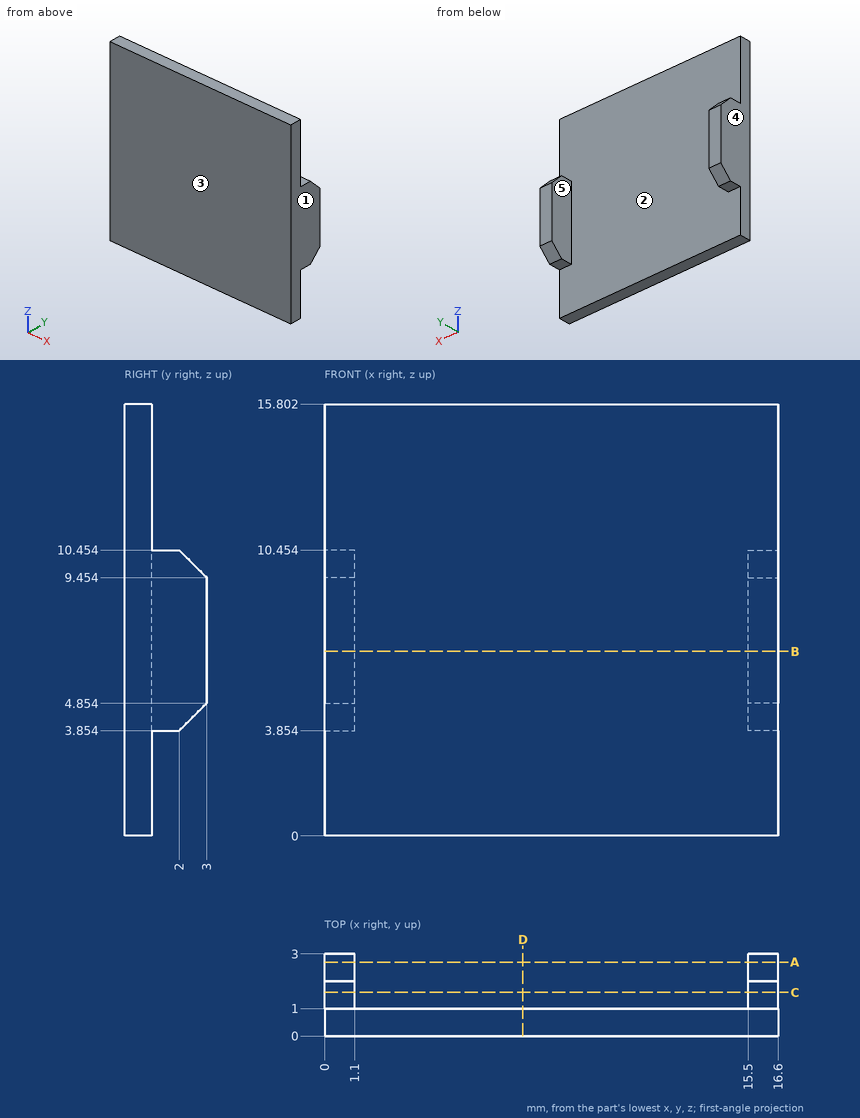
Can you work these out from the drawing? Everything is in mm from the part's minimum corner. A direction names the side the tool comes from. Coordinates: 2 decimals unless noted, no trailing zeros. Loops run counter-clockwise (first coordinate to the right, second up) from the corner with the lowest first, then second, coordinate; pieces in that order, holes last.
1. If we mould it in two halves opening along X, with no side actions, what happens to the marked faces 1, 2 and 3? For each: pulls with the +X half, pulls with the -X half, needs draft (parallel to the pull), parting line crosses it, or undercut.
2. Imagine slicing it at C-C, the plane y = 1.6. Please give me the cut outline in (x, z).
3. Imagine slicing it at B-B, the plane z = 6.75. Please give me the cut outline in (x, y).
4. Imagine slicing it at A-A, the plane y = 2.7. Please give me the cut outline in (x, z).
5. For P1, Ø0.8, axis at x = 16, y = 1.5, coming from the +Z side; P2, Ø0.5, axis at x = 16, y = 1.5, coming from the -Z side, each with a flat end and sliding along its axis, tell me the tip position at first contact or that it passes through.
6. I need wall thicknesses on L1, parallel to X at y = 1.4, z = 4.75; L2, parallel to Y at x = 15.25, z = 5.5; L3, parallel to Z at x = 16.25, y = 2.35 (1 decimal). Which ranges of each line are inside material? Lowest first, please.
7. Imagine slicing it at D-D, the plane x = 7.25. Please give me the cut outline in (y, z), and give its area (3 significant figures).
8. For the marked faces 4 and 5, which set-ups out of +Z, -Z, +X, -X, +Y, -Y let a thin tool reach every point of the face, with its end or its side?
Taken from the geometry:
1. face 1: pulls with the +X half
1. face 2: undercut
1. face 3: needs draft
2. outline: (0, 3.85) - (1.1, 3.85) - (1.1, 10.45) - (0, 10.45) - close; (15.5, 3.85) - (16.6, 3.85) - (16.6, 10.45) - (15.5, 10.45) - close
3. outline: (0, 0) - (16.6, 0) - (16.6, 3) - (15.5, 3) - (15.5, 1) - (1.1, 1) - (1.1, 3) - (0, 3) - close
4. outline: (0, 4.55) - (1.1, 4.55) - (1.1, 9.75) - (0, 9.75) - close; (15.5, 4.55) - (16.6, 4.55) - (16.6, 9.75) - (15.5, 9.75) - close
5. P1: stops at z = 10.45
5. P2: stops at z = 3.85
6. L1: x = 0 to 1.1, 15.5 to 16.6
6. L2: y = 0 to 1
6. L3: z = 4.2 to 10.1
7. outline: (0, 0) - (1, 0) - (1, 15.8) - (0, 15.8) - close
7. area: 15.8 mm2
8. face 4: +Z, -Z, -X, +Y, -Y
8. face 5: +Z, -Z, +Y
